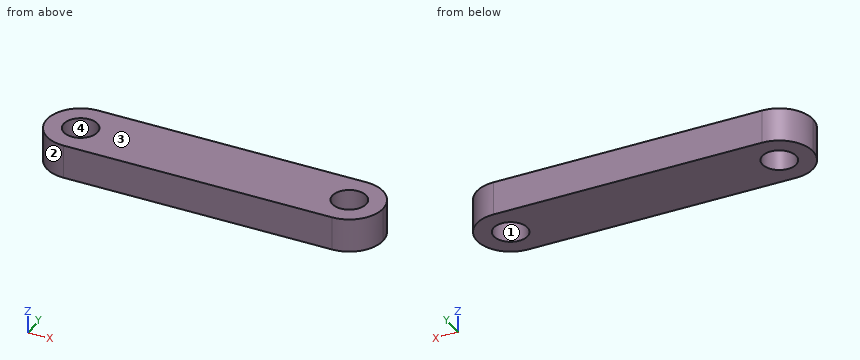
from build123d import *

# Parameters (mm, degrees)
SKETCH1_W           = 100
SKETCH1_H           = 20
BOSS_EXTRUDE1_DEPTH = 10
FILLET1_R           = 10
SKETCH5_R           = 5
CUT_EXTRUDE1_DEPTH  = 103.46950766


with BuildPart() as part:
    # Sketch1 → Boss-Extrude1 (new body)
    with BuildSketch(Plane.XY):
        with Locations((50, 10)):
            Rectangle(SKETCH1_W, SKETCH1_H)
    extrude(amount=BOSS_EXTRUDE1_DEPTH)

    # Fillet1
    fillet1_edges = [part.edges().sort_by_distance(p)[0] for p in [
        (100, 20, 5),
        (100, 0, 5),
        (0, 0, 5),
        (0, 20, 5),
    ]]
    fillet(fillet1_edges, radius=FILLET1_R - 0.0001)  # a hair under: the kernel refuses the full size

    # Sketch5 → Cut-Extrude1 (cut, through all)
    with BuildSketch(Plane.XY.offset(10)):
        with Locations((10, 10)):
            Circle(SKETCH5_R)
        with Locations((90, 10)):
            Circle(SKETCH5_R)
    extrude(amount=-CUT_EXTRUDE1_DEPTH, mode=Mode.SUBTRACT)


solid = part.part
Can you work these out from the model? Positions are in its coordinate system, mm. Face numbers are marked on the shaded views. Give positions to 0.01 mm unless a question says otherwise; leave off trailing zeros. Order: outer loops, then holes, each group sorted by start corner. A loop starts at its lowest first (then second) coordinate and runs counter-clockwise, first axis right, second up. Notation, with made-up numbers: M 47,21 L 94,21 A20 ccw 94,49 Z; hole C 72.5,82 d4. An arc over 180 degrees is marked long. Use one line per item in the form item = value. Start each with the question number.
Item 1: If we section it at C-C (x = 91): Write out the boundary of the cut face in (y, z), then the cut area to 3 significant figures.
Item 2: If we section it at B-B (z = 2.75): State how many separate pieces and enclosed holes the cut face has, then the cut area to 3 significant figures.
Item 3: If we section it at A-A (y = 8): Write out the boundary of the cut face in (x, z).
Item 4: Will these pins go through, and if not, where does the flat tip stop? pin 1 Ø6 at (y, z) = (3, 1.5) entering from -X; pin 2 Ø4 at (y, z) = (16, 6.5) entering from +X; pin 3 Ø3 at (x, y) = (38, 6) entering from -Z; pin 4 Ø3 at (y, z) = (14, 6.5) entering from +X.
Item 5: If I drill on line 1 along Y through (x, z) = (10, 6.5); line 2 along X through (y, z) = (12.5, 8.75); line 3 along X through (y, z) = (13.75, 2.5), over which ranges is the centre line in solid material (lowest first)?
Item 6: We'd pull the mould along X, two halves only. Please class the marked faces 1, 2, 3 and 4: +X half, -X half, draft (parallel to the pull), parting line (faces both ways), or undercut.
Outcome:
q1.outline = M 0.05,0 L 5.1,0 L 5.1,10 L 0.05,10 Z; M 14.9,0 L 19.95,0 L 19.95,10 L 14.9,10 Z
q1.area = 101 mm2
q2.separate_pieces = 1
q2.enclosed_holes = 2
q2.area = 1,760 mm2
q3.outline = M 0.2,0 L 5.42,0 L 5.42,10 L 0.2,10 Z; M 14.58,0 L 85.42,0 L 85.42,10 L 14.58,10 Z; M 94.58,0 L 99.8,0 L 99.8,10 L 94.58,10 Z
q4.pin_1 = 0.83
q4.pin_2 = 99.17
q4.pin_3 = 0
q4.pin_4 = 99.68
q5.line_1 = 0 to 5, 15 to 20
q5.line_2 = 0.32 to 5.67, 14.33 to 85.67, 94.33 to 99.68
q5.line_3 = 0.73 to 6.69, 13.31 to 86.69, 93.31 to 99.27
q6.face_1 = undercut
q6.face_2 = -X half
q6.face_3 = draft
q6.face_4 = undercut
